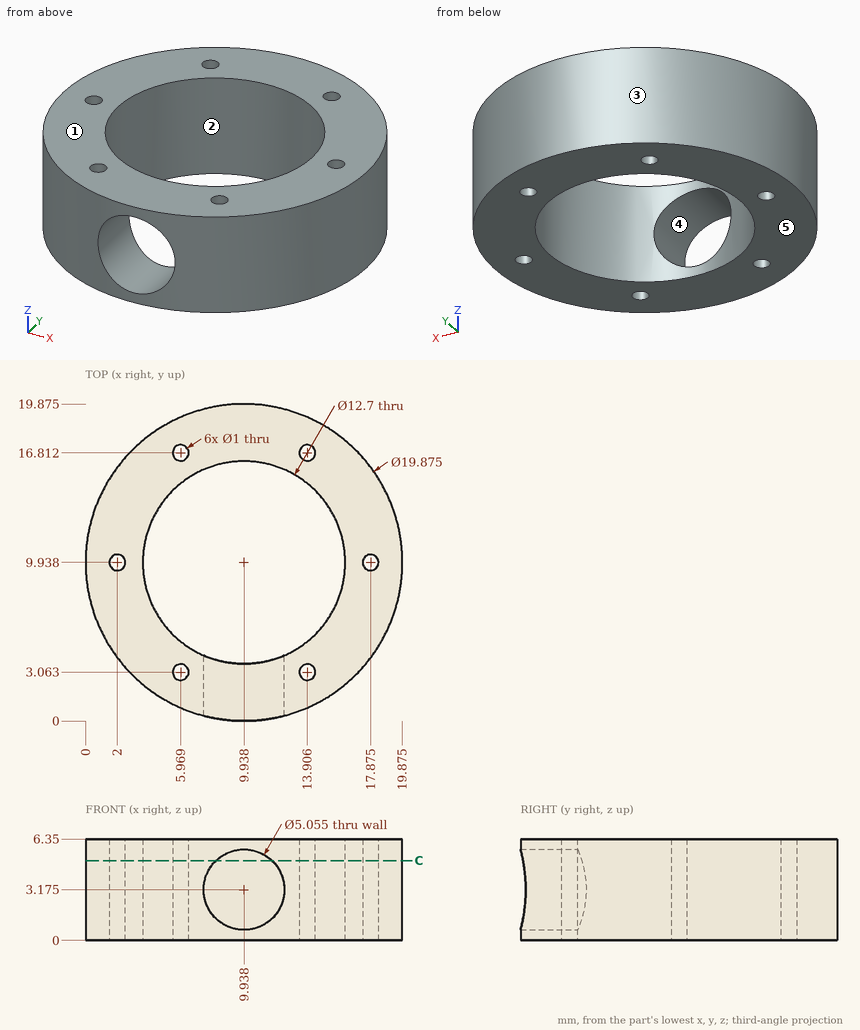
Drawing for the job (mm, zero at the part's lowest x, y, z). A direction names the side the tool comes from. Round coordinates to 2 decimals unless told otherwise and drop trailing zeros. Return JSON: item names as keys, results as strings. Group by question number.
Item 1: 3-axis set-ups, long thin cutter, end or side, ignore diameter. For the marked faces 4 and 5: which of +Z, -Z, +X, -X, +Y, -Y reach the whole face in a straight line?
Item 2: Mould opens along X. For the marked faces 1, 2 and 3 say: +X half, -X half, draft (parallel to the pull), parting line (faces both ways), or undercut.
Item 3: Flat gauge pins, fed straight in: pin 1 Ø1 at (x, z) = (5, 3) entering from -Y (1 decimal); pin 2 Ø1 at (x, y) = (12, 5) entering from -Z. Where does each tip first touch, or does it go through?
Item 4: Probe probe 1 along X at (y, z) = (9, 5.25) (1 decimal); probe 2 along Y at (x, z) = (10.25, 6.25) (1 decimal); probe 3 along X at (y, z) = (10.25, 3.5) (1 decimal). List the from-to ranges inside material, lowest first.
Item 5: Band-saw the part on C-C on z = 5. State how many separate pieces and enclosed holes the cut face has, plus the area to 3 significant figures.
Resolved:
{
 "1": {"face 4": "-Y", "face 5": "-Z, +X, -X, +Y, -Y"},
 "2": {"face 1": "draft", "face 2": "undercut", "face 3": "parting line"},
 "3": {"pin 1": "stops at y = 1", "pin 2": "passes through"},
 "4": {"probe 1": "x = 0 to 3.7, 16.2 to 19.8", "probe 2": "y = 0 to 3.6, 16.3 to 19.9", "probe 3": "x = 0 to 1.6, 2.4 to 3.6, 16.3 to 17.5, 18.3 to 19.9"},
 "5": {"separate pieces": "1", "enclosed holes": "6", "area": "166 mm²"}
}
